Can you work these out from the model? Positions are in its coordinate system, mm. A direction names the side the tool comes from. Give positions to 0.01 mm unless a question says otherwise; leave off trailing zeros. Write each loop counter-clockwise with the first axis right and the second up, starting at its lowest first coordinate (ties: lowest second). Pieces come first, ordered by that corner, then holes. Notation, with made-up numbers: (14.25, -6.5) - (31.25, -6.5) arc R21 ccw to (31.25, -1.5) - close; hole circle Ø2 at (77, -5.75). An arc over 180 degrees is marked (long way). Return JSON: item names as keys, results as strings. Group by question number.
from build123d import *

# Parameters (mm, degrees)
F0_W     = 83.82
F0_H     = 152.6999994
F1_DEPTH = 7.35000054
F2_R     = 5.08
F3_R     = 3.6792614691
F5_DEPTH = 0.762
F4_W     = 12.0734181255
F4_H     = 3.8634948432
F6_DEPTH = 1.27
F8_DEPTH = 0.254


with BuildPart() as f1:
    # F0 (on Top) → F1 (new body)
    with BuildSketch(Plane.XY):
        with Locations((-35.9417264286, 32.7416635112)):
            Rectangle(F0_W, F0_H)
    extrude(amount=F1_DEPTH)

    # F2
    f2_edges = [f1.edges().sort_by_distance(p)[0] for p in [
        (5.968274, -43.608336, 3.675),
        (-77.851726, -43.608336, 3.675),
        (-77.851726, 109.091663, 3.675),
        (5.968274, 109.091663, 3.675),
    ]]
    fillet(f2_edges, radius=F2_R)

    # F3
    f3_edges = [f1.edges().sort_by_distance(p)[0] for p in [
        (5.968274, 32.741664, 7.350001),
        (-77.851726, 32.741664, 7.350001),
    ]]
    fillet(f3_edges, radius=F3_R)

    # F4 (on face) → F5 (join)
    with BuildSketch(Plane.XY.offset(7.35000054)):
        with BuildLine():
            Line((0.8882735714, 105.4124017422), (-72.7717264286, 105.4124017422))
            Line((-72.7717264286, 105.4124017422), (-72.7717264286, -30.1608517766))
            Line((-72.7717264286, -30.1608517766), (-56.5872713923, -30.1608517766))
            Line((-56.5872713923, -30.1608517766), (2.2890121023, -30.1608517766))
            Line((2.2890121023, -30.1608517766), (2.2890121023, 104.0116632112))
            ThreePointArc((2.2890121023, 104.0116632112), (1.8787452853, 105.0021349251), (0.8882735714, 105.4124017422))
        make_face()
    extrude(amount=F5_DEPTH)

    # F4 (on face) → F6 (join)
    with BuildSketch(Plane.XY.offset(7.35000054)):
        with Locations((-36.062461324, -35.7146207243)):
            Rectangle(F4_W, F4_H)
        with BuildLine():
            ThreePointArc((-53.467959375, -35.0449632482), (-54.3815847122, -32.839276568), (-56.5872713923, -31.9256512308))
            Line((-56.5872713923, -31.9256512308), (-56.5872713923, -35.0449632482))
            Line((-56.5872713923, -35.0449632482), (-56.5872713923, -38.1642752656))
            ThreePointArc((-56.5872713923, -38.1642752656), (-54.3815847122, -37.2506499283), (-53.467959375, -35.0449632482))
        make_face()
        with BuildLine():
            Line((-56.5872713923, -35.0449632482), (-56.5872713923, -31.9256512308))
            ThreePointArc((-56.5872713923, -31.9256512308), (-58.7929580725, -32.839276568), (-59.7065834097, -35.0449632482))
            Line((-59.7065834097, -35.0449632482), (-56.5872713923, -35.0449632482))
        make_face()
        with BuildLine():
            Line((-56.5872713923, -35.0449632482), (-59.7065834097, -35.0449632482))
            ThreePointArc((-59.7065834097, -35.0449632482), (-58.7929580725, -37.2506499283), (-56.5872713923, -38.1642752656))
            Line((-56.5872713923, -38.1642752656), (-56.5872713923, -35.0449632482))
        make_face()
        Polygon((-19.8840815574, -33.2999378443), (-23.747574538, -37.1634289622), (-9.7494691825, -37.3968959546), (-13.3644351736, -33.2999378443), align=None)
    extrude(amount=F6_DEPTH)

    # F7 (on face) → F8 (join)
    with BuildSketch(Plane.XY.offset(8.11200054)):
        with BuildLine():
            Line((-37.0942167938, 103.5466420086), (-38.4271452132, 103.5466420086))
            ThreePointArc((-38.4271452132, 103.5466420086), (-38.036739518, 102.6041192844), (-37.0942167938, 102.2137135892))
            Line((-37.0942167938, 102.2137135892), (-37.0942167938, 103.5466420086))
        make_face()
        with BuildLine():
            Line((-35.7612883744, 103.5466420086), (-37.0942167938, 103.5466420086))
            Line((-37.0942167938, 103.5466420086), (-37.0942167938, 102.2137135892))
            ThreePointArc((-37.0942167938, 102.2137135892), (-36.1516940696, 102.6041192844), (-35.7612883744, 103.5466420086))
        make_face()
        with BuildLine():
            ThreePointArc((-35.7612883744, 103.5466420086), (-36.1516940696, 104.4891647328), (-37.0942167938, 104.879570428))
            Line((-37.0942167938, 104.879570428), (-37.0942167938, 103.5466420086))
            Line((-37.0942167938, 103.5466420086), (-35.7612883744, 103.5466420086))
        make_face()
        with BuildLine():
            Line((-37.0942167938, 103.5466420086), (-37.0942167938, 104.879570428))
            ThreePointArc((-37.0942167938, 104.879570428), (-38.036739518, 104.4891647328), (-38.4271452132, 103.5466420086))
            Line((-38.4271452132, 103.5466420086), (-37.0942167938, 103.5466420086))
        make_face()
    extrude(amount=F8_DEPTH)


solid = f1.part
1) Imagine slicing it at A-A, the plane y = -5. Write out the boundary of the cut face in (x, z).
2) Imagine slicing it at B-B, the plane x = -27. Write out the boundary of the cut face in (y, z).
3) On a 3-axis mill with a long thin cutter (end or side, diameter ignored), from which of +Z, -Z, +X, -X, +Y, -Y can I reach the whole of each face in a straight line? I mean faces 1 (the face through (-35.4, -42.5, 6.3)), 2 (the face through (-37, 104, 8.366)), 3 (the face through (-11.53, -35.38, 7.98)). Say none if no direction works.
4) I need wall thicknesses on line 1 along Y through (x, z) = (-65.5, 7.5); line 2 along Z through (x, y) = (-12.5, 32.5); line 3 along Z through (x, y) = (-17, -30.5). Which ranges of each line are inside material? Lowest first, please.
5) We'd pull the mould along Y, two halves only. Please class faces 4 (the face through (-36, -43.608, 2)), 5 (the face through (-36, -36, 8.62)), 6 (the face through (-36.457, 107.985, 6.301)), 7 (the face through (-21.789, -35.205, 7.976)): pulls with the +Y half, pulls with the -Y half, needs draft (parallel to the pull), parting line crosses it, or undercut.
6) Will these pins go through, and if not, where does the flat tip stop? pin 1 Ø0.6 at (y, z) = (-36.5, 8) entering from +X; pin 2 Ø2 at (x, y) = (-36.5, 104) entering from +Z; pin 3 Ø2 at (x, y) = (-17.5, -13) entering from +Z.
Resolved:
{
 "1": {"outline": "(-77.85, 0) - (5.97, 0) - (5.97, 3.67) arc R3.68 ccw to (2.29, 7.35) - (2.29, 8.11) - (-72.77, 8.11) - (-72.77, 7.35) - (-74.17, 7.35) arc R3.68 ccw to (-77.85, 3.67) - close"},
 "2": {"outline": "(-43.61, 0) - (109.09, 0) - (109.09, 3.67) arc R3.68 ccw to (105.41, 7.35) - (105.41, 8.11) - (-30.16, 8.11) - (-30.16, 7.35) - (-39.93, 7.35) arc R3.68 ccw to (-43.61, 3.67) - close"},
 "3": {"face 1": "+Z, +X, -X, -Y", "face 2": "+Z, +X, -X, +Y", "face 3": "+Z, +X"},
 "4": {"line 1": "-30.16 to 105.41", "line 2": "0 to 8.11", "line 3": "0 to 7.35"},
 "5": {"face 4": "pulls with the -Y half", "face 5": "needs draft", "face 6": "pulls with the +Y half", "face 7": "undercut"},
 "6": {"pin 1": "x = -10.28", "pin 2": "z = 8.37", "pin 3": "z = 8.11"}
}
